from build123d import *

# Parameters (mm, degrees)
F0_W     = 150
F0_H     = 150
F0_W_2   = 120
F0_H_2   = 5
F1_DEPTH = 10


with BuildPart() as f1:
    # F0 (on Top) → F1 (new body)
    with BuildSketch(Plane.XY):
        Rectangle(F0_W, F0_H)
        with Locations((0, -47.5)):
            Rectangle(F0_W_2, F0_H_2, mode=Mode.SUBTRACT)
        with Locations((0, -36.944444)):
            Rectangle(F0_W_2, F0_H_2, mode=Mode.SUBTRACT)
        with Locations((0, -26.388889)):
            Rectangle(F0_W_2, F0_H_2, mode=Mode.SUBTRACT)
        with Locations((0, -15.833333)):
            Rectangle(F0_W_2, F0_H_2, mode=Mode.SUBTRACT)
        with Locations((0, -5.277778)):
            Rectangle(F0_W_2, F0_H_2, mode=Mode.SUBTRACT)
        with Locations((0, 5.277778)):
            Rectangle(F0_W_2, F0_H_2, mode=Mode.SUBTRACT)
        with Locations((0, 15.833333)):
            Rectangle(F0_W_2, F0_H_2, mode=Mode.SUBTRACT)
        with Locations((0, 26.388889)):
            Rectangle(F0_W_2, F0_H_2, mode=Mode.SUBTRACT)
        with Locations((0, 36.944444)):
            Rectangle(F0_W_2, F0_H_2, mode=Mode.SUBTRACT)
        with Locations((0, 47.5)):
            Rectangle(F0_W_2, F0_H_2, mode=Mode.SUBTRACT)
    extrude(amount=F1_DEPTH)


solid = f1.part
Verification items for the finished model (mm, model axes). A direction names the side the tool comes from. Round coordinates to 2 decimals unless told otherwise and drop trailing zeros. Order: outer loops, then holes, each group sorted by start corner. A loop starts at its lowest first (then second) coordinate and runs counter-clockwise, first axis right, second up.
1. Section check B-B on x = 7. State how many separate pieces and enclosed holes the cut face has, then the cut area to 3 significant figures.
Final values:
separate pieces: 11
enclosed holes: 0
area: 1,000 mm2
2. Thickness scan on L1, parallel to X at y = 47, z = 1.5. Record the ranges inside material, lowest first.
Final values:
L1: x = -75 to -60, 60 to 75
3. Access from +Z, -Z, +X, -X, +Y, -Y to the whole of each face (thin tool, end or side, straight path). Record for faces 1 (the flat face through (-60, -5, 5)), 2 (the flat face through (-75, -1, 5)).
Final values:
face 1: +Z, -Z
face 2: +Z, -Z, -X, +Y, -Y
4. Release check for a two-part mould opening along Y. For faces 3 (the flat face through (-1, -45, 5)), 4 (the flat face through (75, -1, 5)) record: +Y half, -Y half, draft (parallel to the pull), parting line (faces both ways), or undercut.
Final values:
face 3: undercut
face 4: draft
5. Section check A-A on y = 48. Record the cut outline in (x, z), then the cut area to 3 significant figures.
Final values:
outline: (-75, 0) - (-60, 0) - (-60, 10) - (-75, 10) - close; (60, 0) - (75, 0) - (75, 10) - (60, 10) - close
area: 300 mm2
